from build123d import *

# Parameters (mm, degrees)
F0_W     = 25.4
F0_H     = 25.4
F0_W_2   = 23.8125
F0_H_2   = 23.8125
F1_DEPTH = 279.4
F3_DEPTH = 25.4
F6_DEPTH = 25.4


with BuildPart() as f1:
    # F0 (on Top) → F1 (new body)
    with BuildSketch(Plane.XY):
        Rectangle(F0_W, F0_H)
        Rectangle(F0_W_2, F0_H_2, mode=Mode.SUBTRACT)
    extrude(amount=F1_DEPTH)


with BuildPart() as f3:
    # F2 (on face) → F3 (new body)
    with BuildSketch(Plane.XZ.offset(12.7)):
        Polygon((-117.475, 0), (-12.7, 0), (-12.7, 88.9), (-41.275, 88.9), align=None)
    extrude(amount=-F3_DEPTH)


with BuildPart() as f1_1:
    add(f1.part)

    # F4: union F3
    add(f3.part)

    # F5 (on face) → F6 (cut)
    with BuildSketch(Plane.XZ.offset(12.7)):
        with BuildLine():
            ThreePointArc((6.35, 254), (4.4901280605, 258.4901280605), (0, 260.35))
            ThreePointArc((0, 260.35), (-4.4901280605, 249.5098719395), (6.35, 254))
        make_face()
    extrude(amount=-F6_DEPTH, mode=Mode.SUBTRACT)


solid = f1_1.part
Could you check a few things on this model? Use its own coordinates, in mm. A direction names the side the tool comes from. Coordinates: 2 decimals unless noted, no trailing zeros. Loops run counter-clockwise (first coordinate to the right, second up) from the corner with the lowest first, then second, coordinate; pieces in that order, holes last.
1. Imagine slicing it at B-B (y = 8.5). Please give me the cut outline in (x, z) (3 decimals).
2. For P1, Ø8, axis at x = -57, y = 5.5, coming from the +Z side; P2, Ø10, axis at x = 0, z = 254, coming from the -Y side; P3, Ø14.5, axis at x = 0, z = 254, coming from the +Y side; P4, Ø7, axis at y = 1.5, z = 107, coming from the -X side, each with a flat end and sliding along its axis, tell me the tip position at first contact or that it passes through.
3. We'd pull the mould along X, two halves only. Please class faces 1 (the face through (12.7, 0, 138)), 2 (the face through (-12.7, 0, 183)), 3 (the face through (11.906, 0, 138)): released by +X, released by -X, zero draft, split by the parting line, or undercut.
4. Imagine slicing it at A-A (z = 103). Please give me the cut outline in (x, y), and give its area (3 significant figures).
5. I need wall thicknesses on L1, parallel to Z at x = 0, y = 12.35; L2, parallel to X at y = -12.3, z = 254; L3, parallel to X at y = 6, z = 196.5. Which ranges of each line are inside material? Lowest first, please.
6. For faces 4 (the face through (-10, 12.7, 111)), 5 (the face through (0, 11.906, 138)), 6 (the face through (-27, 0, 88.9)), which set-ups out of +Z, -Z, +X, -X, +Y, -Y let a thin tool reach every point of the face, with its end or its side?
7. Imagine slicing it at D-D (x = -98). Please give me the cut outline in (y, z).
8. Imagine slicing it at C-C (z = 32). Please give me the cut outline in (x, y), and give its area (3 significant figures).
Computed values:
1. outline: (-117.475, 0) - (-11.906, 0) - (-11.906, 279.4) - (-12.7, 279.4) - (-12.7, 88.9) - (-41.275, 88.9) - close; (11.906, 0) - (12.7, 0) - (12.7, 279.4) - (11.906, 279.4) - close
2. P1: stops at z = 75.22
2. P2: passes through
2. P3: stops at y = 12.7
2. P4: stops at x = -12.7
3. face 1: released by +X
3. face 2: released by -X
3. face 3: undercut
4. outline: (-12.7, -12.7) - (12.7, -12.7) - (12.7, 12.7) - (-12.7, 12.7) - close; hole (-11.91, -11.91) - (11.91, -11.91) - (11.91, 11.91) - (-11.91, 11.91) - close
4. area: 78.1 mm2
5. L1: z = 0 to 247.65, 260.35 to 279.4
5. L2: x = -12.7 to -6.35, 6.35 to 12.7
5. L3: x = -12.7 to -11.91, 11.91 to 12.7
6. face 4: +Z, -Z, +X, -X, +Y
6. face 5: +Z, -Z
6. face 6: +Z, -X, +Y, -Y
7. outline: (-12.7, 0) - (12.7, 0) - (12.7, 22.72) - (-12.7, 22.72) - close
8. outline: (-90.05, -12.7) - (12.7, -12.7) - (12.7, 12.7) - (-90.05, 12.7) - close; hole (-11.91, -11.91) - (11.91, -11.91) - (11.91, 11.91) - (-11.91, 11.91) - close
8. area: 2,040 mm2
